Drawing for the job (mm, zero at the part's lowest x, y, z). A direction names the side the tool comes from. Give positions to 0.01 mm unless a question says otherwise; leave off trailing zeros. Loops run counter-clockwise (first coordinate to the right, second up) from the corner with the lowest first, then second, coordinate; pieces in that order, holes last. Notation, with made-up numbers: (14.5, 79) - (21.5, 79) arc R17 cw to (21.5, 86) - close; hole circle Ø3 at (79.5, 54). An arc over 180 degrees is marked (long way). Return JSON: item names as keys, results as strings. Group by question number.
1) Slice it at D-D (y = 3.25). List the corners of the cut face in (x, z), and give its area (3 significant figures).
2) 3-axis set-ups, long thin cutter, end or side, ignore diameter. For the marked faces 1 and 2: which of +Z, -Z, +X, -X, +Y, -Y reach the whole face in a straight line?
3) Drop flat-ended pins along their axis: pin 1 (1.5 mm diameter, centred on x = 29, z = 3.5, fed in from -Y); pin 2 (4 mm diameter, centred on x = 17.5, y = 5.5, fed in from -Z); pin 3 (2 mm diameter, centred on x = 12.5, z = 3.5, fed in from +Y). Give the stop position or say it passes through.
4) Drill centre lines: probe 1 along X at (y, z) = (0.7, 3.5); probe 2 along Z at (x, y) = (7.5, 3.25); probe 3 along Y at (x, z) = (16.5, 2.5). Where is each one in solid material? Low to high. Write a range as from..to.
5) Slice it at C-C (y = 1.5). List the corners of the cut face in (x, z).
6) Slice it at B-B (x = 29). List the corners of the cut face in (y, z), and give its area (3 significant figures).
7) Slice it at A-A (z = 3.5). List the corners of the cut face in (x, y), and give its area (3 significant figures).
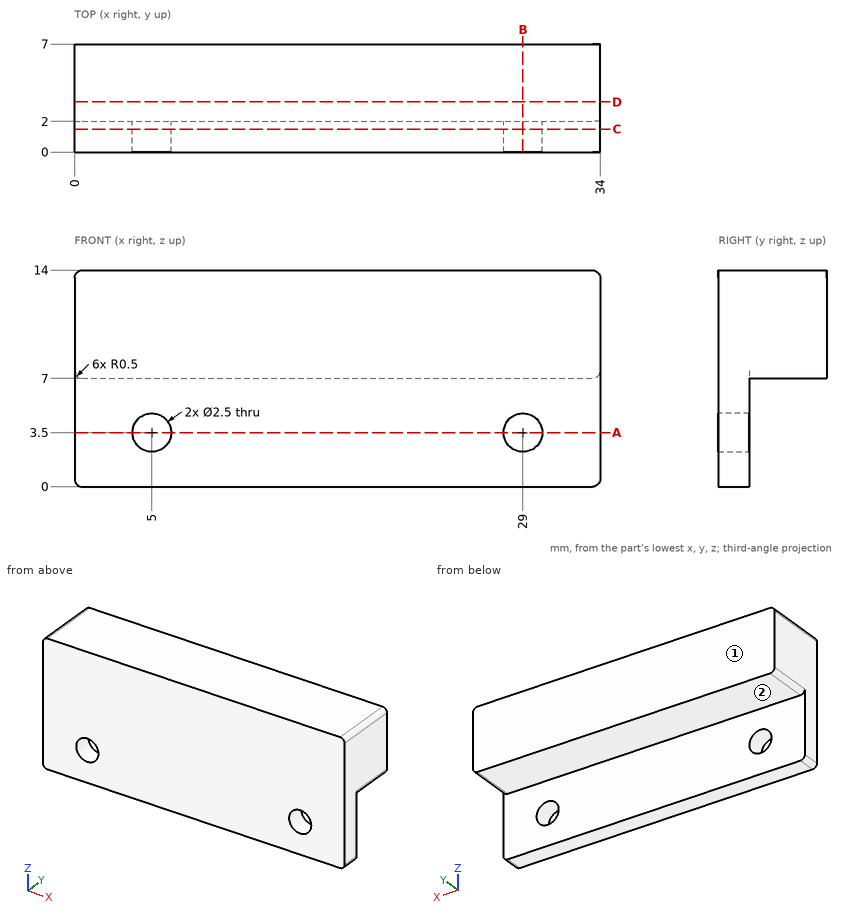
Results:
{
 "1": {"outline": "(0, 7.5) arc R0.5 ccw to (0.5, 7) - (33.5, 7) arc R0.5 ccw to (34, 7.5) - (34, 13.5) arc R0.5 ccw to (33.5, 14) - (0.5, 14) arc R0.5 ccw to (0, 13.5) - close", "area": "238 mm2"},
 "2": {"face 1": "+Z, -Z, +X, -X, +Y", "face 2": "-Z, +X, -X, +Y"},
 "3": {"pin 1": "through", "pin 2": "z = 7", "pin 3": "y = 2"},
 "4": {"probe 1": "0..3.75, 6.25..27.75, 30.25..34", "probe 2": "7..14", "probe 3": "0..2"},
 "5": {"outline": "(0, 0.5) arc R0.5 ccw to (0.5, 0) - (33.5, 0) arc R0.5 ccw to (34, 0.5) - (34, 13.5) arc R0.5 ccw to (33.5, 14) - (0.5, 14) arc R0.5 ccw to (0, 13.5) - close; hole circle Ø2.5 at (5, 3.5); hole circle Ø2.5 at (29, 3.5)"},
 "6": {"outline": "(0, 0) - (2, 0) - (2, 2.25) - (0, 2.25) - close; (0, 4.75) - (2, 4.75) - (2, 7) - (7, 7) - (7, 14) - (0, 14) - close", "area": "58.0 mm2"},
 "7": {"outline": "(0, 0) - (3.75, 0) - (3.75, 2) - (0, 2) - close; (6.25, 0) - (27.75, 0) - (27.75, 2) - (6.25, 2) - close; (30.25, 0) - (34, 0) - (34, 2) - (30.25, 2) - close", "area": "58.0 mm2"}
}
